Build history of the part. All positions in model axes, mm. A direction names the side the tool comes from. Give positions to 0.01 mm unless a question says otherwise; leave off trailing zeros. Order: outer loops, then holes, each group sorted by start corner. A loop starts at its lowest first (then second) coordinate and runs counter-clockwise, first axis right, second up. Notation, with made-up numbers: M -5,-35 L 34,-35 A11 cw 34,-28 Z; hole C 85.25,-32.75 d6. An arc over 180 degrees is marked long. Answer as CSV lines item,"result".
from build123d import *

# Parameters (mm, degrees)
F1_DEPTH = 350
F2_W     = 12.5
F2_H     = 25
F3_DEPTH = 262.501
F5_DEPTH = 25.001


with BuildPart() as f1:
    # F0 (on Top) → F1 (new body)
    with BuildSketch(Plane.XY):
        with BuildLine():
            Line((0, 25), (0, 0))
            Line((0, 0), (250, 0))
            ThreePointArc((250, 0), (262.5, 12.5), (250, 25))
            Line((250, 25), (0, 25))
        make_face()
    extrude(amount=F1_DEPTH)

    # F2 (on face) → F3 (cut, through all)
    with BuildSketch(Plane(origin=(0, 0, 0), x_dir=(0, -1, 0), z_dir=(-1, 0, 0))):
        with Locations((-18.75, 287.5)):
            Rectangle(F2_W, F2_H)
    extrude(amount=-F3_DEPTH, mode=Mode.SUBTRACT)

    # F4 (on face) → F5 (cut, through all)
    with BuildSketch(Plane.XZ):
        Polygon((250, 0), (250, 225.185185), (60, 0), align=None)
        Polygon((262.5, 0), (262.5, 240), (250, 225.185185), (250, 0), align=None)
    extrude(amount=-F5_DEPTH, mode=Mode.SUBTRACT)


solid = f1.part
Item 1: Probe line 1 along Z through (x, y) = (56, 15.25); line 2 along Y through (x, z) = (139.5, 287); line 3 along Z through (x, y) = (152, 16.5). List the from-to ranges inside material, lowest first. Write a range as from..to.
Geometry says:
line 1,"z = 0..275, 300..350"
line 2,"y = 0..12.5"
line 3,"z = 109.04..275, 300..350"
Item 2: Band-saw the part on C-C (z = 168). Give the cut face in (x, y).
Geometry says:
outline,"M 0,0 L 201.75,0 L 201.75,25 L 0,25 Z"
Item 3: Band-saw the part on A-A (x = 18). Give the cut face in (y, z), and give its area (3 significant figures).
Geometry says:
outline,"M 0,0 L 25,0 L 25,275 L 12.5,275 L 12.5,300 L 25,300 L 25,350 L 0,350 Z"
area,"8,440 mm2"
Item 4: Drop flat-ended pins along their axis: pin 1 (14 mm diameter, centred on x = 155.5, y = 18.5, fed in from -Z); pin 2 (4 mm diameter, centred on y = 3.5, z = 190.5, fed in from +X); pin 3 (12 mm diameter, centred on y = 8, z = 161, fed in from +X). Give the stop position or say it passes through.
Geometry says:
pin 1,"stops at z = 104.89"
pin 2,"stops at x = 222.42"
pin 3,"stops at x = 200.91"
Item 5: Band-saw the part on D-D (x = 98.5). Give the cut face in (y, z), and give its area (3 significant figures).
Geometry says:
outline,"M 0,45.63 L 25,45.63 L 25,275 L 12.5,275 L 12.5,300 L 25,300 L 25,350 L 0,350 Z"
area,"7,300 mm2"
Item 6: Pull direction Z, two halves, no side cores. Call faces 1 (the flat face through (129, 19, 300)), 2 (the flat face through (129, 13, 350)), 3 (the flat face through (95, 0, 211)), 4 (the flat face through (129, 12.5, 287)): released by +Z, released by -Z, zero draft, split by the parting line, or undercut.
Geometry says:
face 1,"undercut"
face 2,"released by +Z"
face 3,"zero draft"
face 4,"undercut"
Item 7: 3-axis set-ups, long thin cutter, end or side, ignore diameter. For faces 5 (the flat face through (127, 25, 325)), 6 (the flat face through (129, 19, 275)): which of +Z, -Z, +X, -X, +Y, -Y reach the whole face in a straight line?
Geometry says:
face 5,"+Z, -Z, +X, -X, +Y"
face 6,"+X, -X, +Y"
Item 8: Band-saw the part on B-B (y = 7.25). Give the cut face in (x, z), and give its area (3 significant figures).
Geometry says:
outline,"M 0,0 L 60,0 L 261.34,238.63 L 261.34,350 L 0,350 Z"
area,"67,400 mm2"
